Verification items for the finished model (mm, model axes). A direction names the side the tool comes from. Round coordinates to 2 decimals unless told otherwise and drop trailing zeros. Loops run counter-clockwise (first coordinate to the right, second up) from the corner with the lowest first, then second, coordinate; pieces in that order, holes last. Notation, with made-up numbers: M -21,72 L 10,72 A28 ccw 10,103 Z; hole C 20.5,32 d6. An arc over 180 degrees is marked long. Answer as CSV lines item,"result".
Autodesk Inventor part; units mm, degrees
ref_plane "YZ Plane" through (0, 0, 0) normal (1, 0, 0) x (0, 1, 0)
ref_plane "XZ Plane" through (0, 0, 0) normal (0, 1, 0) x (-1, 0, 0)
ref_plane "XY Plane" through (0, 0, 0) normal (0, 0, 1) x (1, 0, 0)
sketch "Sketch1" plane through (0, 0, 0) normal (0, 0, 1) x (1, 0, 0)
  line L0 (0, 0) -> (711.2, 0)
  line L1 (711.2, 0) -> (711.2, 558.8)
  line L2 (711.2, 558.8) -> (0, 558.8)
  line L3 (0, 558.8) -> (0, 0)
  line L4 (50.8, 508) -> (660.4, 508)
  line L5 (660.4, 508) -> (660.4, 50.8)
  line L6 (660.4, 50.8) -> (50.8, 50.8)
  line L7 (50.8, 50.8) -> (50.8, 508)
  line L8 (609.6, 457.2) -> (101.6, 457.2)
  line L9 (101.6, 457.2) -> (101.6, 101.6)
  line L10 (101.6, 101.6) -> (609.6, 101.6)
  line L11 (609.6, 101.6) -> (609.6, 457.2)
  line L12 (152.4, 406.4) -> (558.8, 406.4)
  line L13 (558.8, 406.4) -> (558.8, 152.4)
  line L14 (558.8, 152.4) -> (152.4, 152.4)
  line L15 (152.4, 152.4) -> (152.4, 406.4)
  dimension "d2" = 50.8
  dimension "d3" = 50.8
  dimension "d4" = 50.8
  dimension "d9" = 457.2
  dimension "d10" = 609.6
extrude "Extrusion1" add sketch "Sketch1" along normal blind 4.7752 contours L3 L2 L1 L0 | L4 L5 L6 L7 | L11 L10 L9 L8
extrude "Extrusion2" add sketch "Sketch1" along normal blind 7.9375 contours L4 L5 L6 L7
properties part number "square"
1) Section check D-D (x = 651). Record the cut outline in (y, z).
Here are the results:
outline,"M 0,0 L 558.8,0 L 558.8,4.78 L 508,4.78 L 508,7.94 L 50.8,7.94 L 50.8,4.78 L 0,4.78 Z"
2) Section check C-C (y = 165.5). Record the cut outline in (x, z).
Here are the results:
outline,"M 0,0 L 152.4,0 L 152.4,4.78 L 101.6,4.78 L 101.6,7.94 L 50.8,7.94 L 50.8,4.78 L 0,4.78 Z; M 558.8,0 L 711.2,0 L 711.2,4.78 L 660.4,4.78 L 660.4,7.94 L 609.6,7.94 L 609.6,4.78 L 558.8,4.78 Z"
3) Go/stop test with flat-tipped pins: pin 1 (1.6 mm diameter, centred on x = 267, z = 6, fed in from +Y); pin 2 (1.6 mm diameter, centred on y = 226.5, z = 6, fed in from +X); pin 3 (2 mm diameter, centred on x = 188, y = 119, fed in from +Z). Record where each tip stops, or that it passes through.
Here are the results:
pin 1,"stops at y = 508"
pin 2,"stops at x = 660.4"
pin 3,"stops at z = 4.78"
4) Material ranges on probe 1 along Y at (x, z) = (345, 3); probe 2 along Y at (x, z) = (159, 7.5); probe 3 along X at (y, z) = (318, 6), recorded low to high.
Here are the results:
probe 1,"y = 0 to 152.4, 406.4 to 558.8"
probe 2,"y = 50.8 to 101.6, 457.2 to 508"
probe 3,"x = 50.8 to 101.6, 609.6 to 660.4"
5) Section check A-A (x = 505). Record the cut outline in (y, z).
Here are the results:
outline,"M 0,0 L 152.4,0 L 152.4,4.78 L 101.6,4.78 L 101.6,7.94 L 50.8,7.94 L 50.8,4.78 L 0,4.78 Z; M 406.4,0 L 558.8,0 L 558.8,4.78 L 508,4.78 L 508,7.94 L 457.2,7.94 L 457.2,4.78 L 406.4,4.78 Z"
6) Set-up check for faces 1 (the flat face through (352, 440, 4.775)), 2 (the flat face through (351, 486, 7.938)): record each of +Z, -Z, +X, -X, +Y, -Y from which the full face is reachable in a straight line by a thin tool's end or side.
Here are the results:
face 1,"+Z"
face 2,"+Z, +X, -X, +Y, -Y"
7) Section check B-B (z = 1.5). Record the cut outline in (x, y), plus the area to 3 significant figures.
Here are the results:
outline,"M 0,0 L 711.2,0 L 711.2,558.8 L 0,558.8 Z; hole M 152.4,152.4 L 558.8,152.4 L 558.8,406.4 L 152.4,406.4 Z"
area,"294,000 mm^2"
